Source: three-view drawing plus pictorial views. Frame: mm from the lowest corner of the part. A direction names the side the tool comes from. Round coordinates to 2 decimals unless told otherwise and drop trailing zeros. Order: outer loops, then holes, each group sorted by start corner. A loop starts at its lowest first (then second) coordinate and runs counter-clockwise, first axis right, second up. Notation, with made-up numbers: (39, 79.5) -> (53, 79.5) arc R26 ccw to (53, 95.5) -> close; hole circle Ø5 at (-15, 53.5). An arc over 180 degrees is marked (long way). Use a Markdown table: item, result.
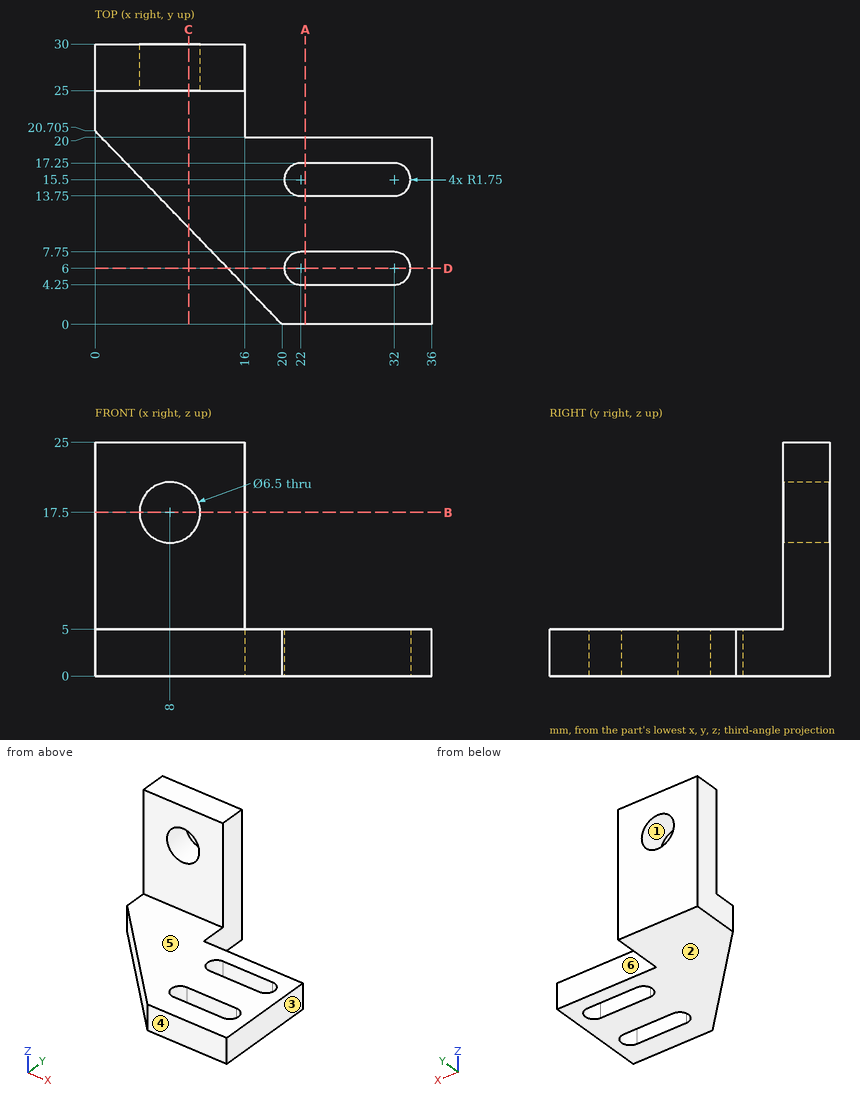
1) Cut plane D-D on y = 6. Return loops of the section in (x, z).
Results found:
| item | result |
|---|---|
| outline | (14.2, 0) -> (20.25, 0) -> (20.25, 5) -> (14.2, 5) -> close; (33.75, 0) -> (36, 0) -> (36, 5) -> (33.75, 5) -> close |
2) Pull-direction query (X, two-part tool) for the marked faces 1, 2 and 3; classes: +X half, -X half, draft (parallel to the pull), parting line (faces both ways), or undercut.
Results found:
| item | result |
|---|---|
| face 1 | undercut |
| face 2 | draft |
| face 3 | +X half |
3) Pin query (flat end, axial travel): pin 1 Ø3 at (y, z) = (24, 16) entering from +X; pin 2 Ø1.5 at (x, z) = (27, 3.5) entering from +Y; pin 3 Ø7.5 at (x, y) = (17, 6.5) entering from +Z. Return the tip coordinate at first contact, or that it passes through.
Results found:
| item | result |
|---|---|
| pin 1 | stops at x = 16 |
| pin 2 | stops at y = 20 |
| pin 3 | stops at z = 5 |
4) Line query: L1, parallel to Y at x = 21, z = 4.25; L2, parallel to Z at x = 8, y = 26.7; L3, parallel to X at y = 27.25, z = 8. Output: solid intervals per line, ascending. Write a range as [from, to].
Results found:
| item | result |
|---|---|
| L1 | y = [0, 4.56], [7.44, 14.06], [16.94, 20] |
| L2 | z = [0, 14.25], [20.75, 25] |
| L3 | x = [0, 16] |
5) Cut plane C-C on x = 10. Return loops of the section in (y, z).
Results found:
| item | result |
|---|---|
| outline | (10.35, 0) -> (30, 0) -> (30, 14.94) -> (25, 14.94) -> (25, 5) -> (10.35, 5) -> close; (25, 20.06) -> (30, 20.06) -> (30, 25) -> (25, 25) -> close |
6) Cut plane A-A on x = 22.5. Return loops of the section in (y, z), and give its area (3 significant figures).
Results found:
| item | result |
|---|---|
| outline | (0, 0) -> (4.25, 0) -> (4.25, 5) -> (0, 5) -> close; (7.75, 0) -> (13.75, 0) -> (13.75, 5) -> (7.75, 5) -> close; (17.25, 0) -> (20, 0) -> (20, 5) -> (17.25, 5) -> close |
| area | 65.0 mm² |
7) Set-up query: the marked faces 4, 5 and 6. Return all of +Z, -Z, +X, -X, +Y, -Y with unobstructed straight access to the full face (end or side cutting, diameter ignored); none if empty.
Results found:
| item | result |
|---|---|
| face 4 | +Z, -Z, +X, -X, -Y |
| face 5 | +Z, +X, -X, -Y |
| face 6 | +Z, -Z, +X, +Y |
8) Cut plane B-B on z = 17.5. Return loops of the section in (x, y), and give its area (3 significant figures).
Results found:
| item | result |
|---|---|
| outline | (0, 25) -> (4.75, 25) -> (4.75, 30) -> (0, 30) -> close; (11.25, 25) -> (16, 25) -> (16, 30) -> (11.25, 30) -> close |
| area | 47.5 mm² |
